Here's how the part is built. I have some questions about the finished solid (model axes, mm). A direction names the side the tool comes from. Give positions to 0.01 mm unless a question says otherwise; leave off trailing zeros. Loops run counter-clockwise (first coordinate to the right, second up) from the corner with the lowest first, then second, coordinate; pieces in that order, holes last.
Q1. If we section it at C-C (z = -7): Please give me the cut outline in (x, y).
Q2. For faces 1 (the face through (38, -71, -14.605)), 2 (the face through (42.774, -67.09, 15.231)), 3 (the face through (35, -64, -15.875)), which set-ups out of +Z, -Z, +X, -X, +Y, -Y let a thin tool reach every point of the face, with its end or its side?
Q3. We'd pull the mould along X, two halves only. Please class faces 4 (the face through (27, -83, -15.875)), 5 (the face through (-75.587, 57.958, -0.204)), 6 (the face through (32.96, 63.38, -0.2)): +X half, -X half, draft (parallel to the pull), parting line (faces both ways), or undercut.
Q4. I need wall thicknesses on line 1 (X direction, y = 0.5, z = 12.5); line 2 (Y direction, x = 0, z = 15.2); line 3 (Y direction, x = 0, z = -15.3). Which ranges of each line are inside material? Lowest first, please.
Q5. Will these pins go through, and if not, where does the flat tip stop? P1, Ø12, axis at y = 34, z = -6.5, coming from the +X side; P2, Ø1.5, axis at x = 27.5, z = 11, coming from the -Y side; P3, Ø1, axis at x = 27, z = 3.5, coming from the +Y side.
Autodesk Inventor part; units mm, degrees
ref_plane "YZ Plane" through (0, 0, 0) normal (1, 0, 0) x (0, 1, 0)
ref_plane "XZ Plane" through (0, 0, 0) normal (0, 1, 0) x (-1, 0, 0)
ref_plane "XY Plane" through (0, 0, 0) normal (0, 0, 1) x (1, 0, 0)
sketch "Sketch1" plane through (0, 0, 0) normal (0, 0, 1) x (1, 0, 0)
  circle A0 centre (0, 0) radius 7.1437
  circle A1 centre (0, 0) radius 9.525
  circle A2 centre (0, 0) radius 7.9566
  circle A3 centre (0, 0) radius 8.7122
  dimension "d0" = 14.2875
  dimension "d1" = 19.05
  dimension "d2" = 0.8128
  dimension "d3" = 0.8128
extrude "Extrusion1" add sketch "Sketch1" along normal mid plane 3.175
fillet "Fillet1" radius 0.127 2 edges at (-9.525, 0, 1.5875) (-9.525, 0, -1.5875)
chamfer "Chamfer1" distance 0.127 angle 45 2 edges at (-7.1437, 0, 1.5875) (-7.1437, 0, -1.5875)
sketch "Sketch2" plane through (0, 0, 0) normal (0, 0, 1) x (1, 0, 0)
  circle A0 centre (0, 0) radius 8.7122
  circle A1 centre (0, 0) radius 7.9566
extrude "Extrusion2" add sketch "Sketch2" along normal mid plane 2.921
scale "Scale1" factors (10, 10, 10) then translate (0, 0, 0) bodies 1
properties part number "front hub bearing"
Check sheet entries:
1. outline: circle Ø190.5 at (0, 0); hole circle Ø142.87 at (0, 0)
2. face 1: -Z
2. face 2: +Z
2. face 3: -Z, +X, -X, +Y, -Y
3. face 4: draft
3. face 5: parting line
3. face 6: undercut
4. line 1: x = -95.25 to -71.44, 71.44 to 95.25
4. line 2: y = -95.1 to -87.12, -79.57 to -72.03, 72.03 to 79.57, 87.12 to 95.1
4. line 3: y = -95.04 to -87.12, -79.57 to -72.13, 72.13 to 79.57, 87.12 to 95.04
5. P1: stops at x = 91.04
5. P2: stops at y = -91.42
5. P3: stops at y = 91.49
